from build123d import *

# Parameters (mm, degrees)
SKETCH1_R           = 4.250000000000005
SKETCH1_R_2         = 4.250000000000013
SKETCH1_R_3         = 4.2500000000000036
BOSS_EXTRUDE1_DEPTH = 7
FILLET2_R           = 6.5
SKETCH4_R           = 7
BOSS_EXTRUDE3_DEPTH = 26
SKETCH5_R           = 7.75
BOSS_EXTRUDE4_DEPTH = 6
FILLET3_R           = 6.5
FILLET4_R           = 6.5
FILLET5_R           = 6.5


with BuildPart() as part:
    # Sketch1 → Boss-Extrude1 (new body)
    with BuildSketch(Plane(origin=(0, 0, 0), x_dir=(1, 0, 0), z_dir=(0, 1, 0))):
        Polygon((-27, 27), (27, 27), (27.000000000000007, -27), (-26.999999999999993, -27), align=None)
        with Locations(Location((-20.329319959113246, 20.329319959113246, 0), (0, 0, 270))):
            Circle(SKETCH1_R, mode=Mode.SUBTRACT)
        with Locations(Location((20.32931995911324, -20.329319959113246, 0), (0, 0, 90))):
            Circle(SKETCH1_R_2, mode=Mode.SUBTRACT)
        with Locations(Location((-20.329319959113224, -20.329319959113246, 0), (0, 0, 270))):
            Circle(SKETCH1_R_2, mode=Mode.SUBTRACT)
        with Locations(Location((20.329319959113246, 20.329319959113253, 0), (0, 0, 90))):
            Circle(SKETCH1_R_3, mode=Mode.SUBTRACT)
    extrude(amount=BOSS_EXTRUDE1_DEPTH)

    # Fillet2
    fillet2_edges = [part.edges().sort_by_distance(p)[0] for p in [
        (27.000000000000007, 3.5, 27),
        (-26.999999999999993, 3.5, 27),
        (-27, 3.5, -27),
        (27, 3.5, -27),
    ]]
    fillet(fillet2_edges, radius=FILLET2_R)

    # Sketch4 → Boss-Extrude3 (add)
    with BuildSketch(Plane(origin=(0, 7, 0), x_dir=(1, 0, 0), z_dir=(0, 1, 0))):
        with Locations(Location((0, 0, 0), (0, 0, 90))):
            Circle(SKETCH4_R)
    extrude(amount=BOSS_EXTRUDE3_DEPTH)

    # Sketch5 → Boss-Extrude4 (add)
    with BuildSketch(Plane(origin=(0, 33, 0), x_dir=(1, 0, 0), z_dir=(0, 1, 0))):
        with Locations(Location((0, 0, 0), (0, 0, 270))):
            Circle(SKETCH5_R)
    extrude(amount=BOSS_EXTRUDE4_DEPTH)

    # Sketch6 → Cut-Revolve1 (revolve, cut)
    with BuildSketch(Plane.XY, mode=Mode.PRIVATE) as cut_revolve1_sk:
        Polygon((6.8958692457127615, 39.84698008319777), (7.935722009021632, 31.389012156149754), (8.514556179291803, 31.389012156149754), (8.514556179291803, 39.84698008319777), align=None)
    revolve(cut_revolve1_sk.sketch.rotate(Axis((0, 39, 0), (0, -1, 0)), 90), axis=Axis((0, 39, 0), (0, -1, 0)), mode=Mode.SUBTRACT)

    # Fillet3
    fillet3_edges = [part.edges().sort_by_distance(p)[0] for p in [
        (-1.29e-15, 7, 7),
    ]]
    fillet(fillet3_edges, radius=FILLET3_R)

    # Sketch7 → Cut-Revolve2 (revolve, cut)
    with BuildSketch(Plane.XY, mode=Mode.PRIVATE) as cut_revolve2_sk:
        Polygon((4.999999999999997, 41.673662522697256), (5.000000000000003, 4.999999999999999), (14.500000000000009, 5), (14.50000000000001, 1.128e-14), (0, -2.109667236724723), (1.73e-15, 41.673662522697256), align=None)
    revolve(cut_revolve2_sk.sketch.rotate(Axis((1.73e-15, 41.673662522697256, 0), (-4e-17, -1, 0)), 180), axis=Axis((1.73e-15, 41.673662522697256, 0), (-4e-17, -1, 0)), mode=Mode.SUBTRACT)

    # Fillet4
    fillet4_edges = [part.edges().sort_by_distance(p)[0] for p in [
        (5.000000000000003, 5, -1.22e-15),
    ]]
    fillet(fillet4_edges, radius=FILLET4_R)

    # Fillet5
    # the kernel refuses this fillet: 6.5 mm, written as the material it adds along each edge
    with BuildSketch(Plane(origin=(2.8e-16, 5, 0), x_dir=(-1, 6e-17, 1.2e-16), z_dir=(1.2e-16, 0, 1))) as fillet5_piece_1:
        with BuildLine():
            CenterArc((8.084264649295068, 6.043235308880427), FILLET5_R, 285.23323327747323, 65.5309787307709)
            Line((14.500000000001535, 4.999999999999738), (15.141573535072181, 4.895676469111669))
            ThreePointArc((15.141573535072181, 4.895676469111669), (15.15000000000001, 2.499999999999869), (15.15000000000001, 4e-17))
            Line((15.15000000000001, 4e-17), (14.500000000000009, -0.6500000000000004))
            ThreePointArc((14.500000000000009, -0.6500000000000004), (11.499999999999995, -0.6500000000000006), (9.962919092182778, -0.8555441110038083))
            Line((9.962919092182778, -0.8555441110038083), (9.792132324647532, -0.22838234555978715))
        make_face()
    revolve(axis=Axis((2.8e-16, 5, 0), (-4e-17, -1, 0)))


solid = part.part
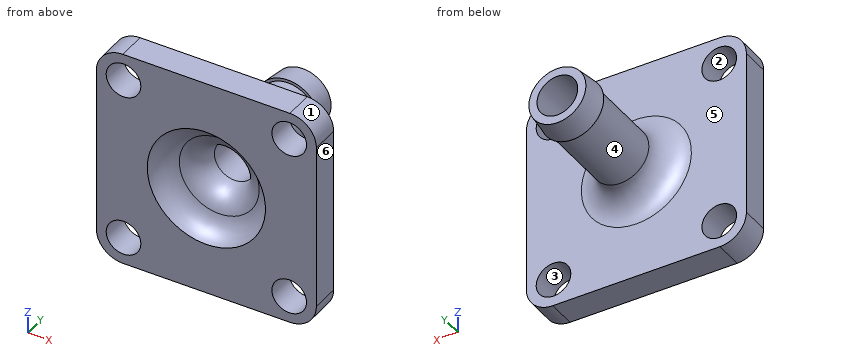
Verification items for the finished model (mm, model axes). Face numbers are marked on the shaded views. A direction names the side the tool comes from. Round coordinates to 2 decimals unless told otherwise and drop trailing zeros. Loops run counter-clockwise (first coordinate to the right, second up) from the corner with the lowest first, then second, coordinate; pieces in that order, holes last. Notation, with made-up numbers: (-28.75, -38) - (-19.75, -38) arc R30 cw to (-19.75, -7) - close; hole circle Ø4 at (-34.75, 2). An arc over 180 degrees is marked (long way). Use one line per item in the form item = value.
1. Section check B-B on y = 4.5. Record the cut outline in (x, z).
A:
outline = (-27, -20.5) arc R6.5 ccw to (-20.5, -27) - (20.5, -27) arc R6.5 ccw to (27, -20.5) - (27, 20.5) arc R6.5 ccw to (20.5, 27) - (-20.5, 27) arc R6.5 ccw to (-27, 20.5) - close; hole circle Ø8.5 at (-20.33, -20.33); hole circle Ø8.5 at (-20.33, 20.33); hole circle Ø22.96 at (0, 0); hole circle Ø8.5 at (20.33, -20.33); hole circle Ø8.5 at (20.33, 20.33)
2. Draft check along X on the marked faces 1, 2, 3 and 4. Enter one of: pulls with the +X half, pulls with the -X half, needs draft (parallel to the pull), parting line crosses it, or undercut.
A:
face_1 = pulls with the +X half
face_2 = undercut
face_3 = undercut
face_4 = parting line crosses it
3. Scan lines: probe 1 along Y at (x, z) = (19.5, 0.5); probe 2 along Z at (x, y) = (-7.5, 2.5); probe 3 along Z at (x, y) = (-2, 21). Record each from-to range of solid material in increasing order.
A:
probe_1 = 0 to 7
probe_2 = -27 to -11.27, 11.27 to 27
probe_3 = -6.71 to -4.58, 4.58 to 6.71
4. Access from +Z, -Z, +X, -X, +Y, -Y to the whole of each face (thin tool, end or side, straight path). Record for the marked faces 5 and 6.
A:
face_5 = +Y
face_6 = +Z, -Z, +X, +Y, -Y
5. Section check A-A on z = -23. Record the cut outline in (x, y), and give its area (3 significant figures).
A:
outline = (-26.5, 0) - (-23.64, 0) - (-23.64, 7) - (-26.5, 7) - close; (-17.02, 0) - (17.02, 0) - (17.02, 7) - (-17.02, 7) - close; (23.64, 0) - (26.5, 0) - (26.5, 7) - (23.64, 7) - close
area = 278 mm²
6. Section check C-C on y = 31. Record the cut outline in (x, z).
A:
outline = circle Ø14 at (0, 0); hole circle Ø10 at (0, 0)
7. Section check D-D on z = 21.5. Record the cut outline in (x, y).
A:
outline = (-26.92, 0) - (-24.41, 0) - (-24.41, 7) - (-26.92, 7) - close; (-16.24, 0) - (16.24, 0) - (16.24, 7) - (-16.24, 7) - close; (24.41, 0) - (26.92, 0) - (26.92, 7) - (24.41, 7) - close
8. Gauge pin test, flat ends, axial feed: pin 1 Ø6 at (x, z) = (15.5, -12) entering from +Y; pin 2 Ø7.5 at (x, z) = (-20.33, -20.33) entering from +Y. Record the tip position at first contact, or that the pin passes through.
A:
pin_1 = 7
pin_2 = through
